Could you check a few things on this model? Use its own coordinates, in mm. Give positions to 0.01 mm unless a question says otherwise; leave off trailing zeros. Loops run counter-clockwise (first coordinate to the right, second up) from the corner with the lowest first, then second, coordinate; pieces in that order, holes last. Notation, with made-up numbers: (84, 84.25) - (94, 84.25) arc R20 cw to (94, 122.25) - close; hole circle Ø10 at (2, 77.5). An arc over 180 degrees is marked (long way). Answer in a Markdown table with one row per item. Add a question column.
```python
from build123d import *

# Parameters (mm, degrees)
SKETCH1_W           = 185
SKETCH1_H           = 84
SKETCH1_R           = 2.25
BOSS_EXTRUDE1_DEPTH = 5
SKETCH2_W           = 185
SKETCH2_H           = 79
SKETCH2_R           = 2.25
BOSS_EXTRUDE2_DEPTH = 3
CHAMFER1_SIZE       = 8
CHAMFER3_SIZE       = 3
SKETCH3_W           = 7.071067812
SKETCH3_H           = 2.6
CUT_EXTRUDE1_DEPTH  = 221.270985121
SKETCH4_R           = 29
SKETCH4_R_2         = 1.75
CUT_EXTRUDE2_DEPTH  = 204.334699449


with BuildPart() as part:
    # Sketch1 → Boss-Extrude1 (new body)
    with BuildSketch(Plane.XY):
        with Locations((92.5, 42)):
            Rectangle(SKETCH1_W, SKETCH1_H)
        with Locations((15, 9)):
            Circle(SKETCH1_R, mode=Mode.SUBTRACT)
        with Locations(Location((170, 9, 0), (0, 0, 180))):
            Circle(SKETCH1_R, mode=Mode.SUBTRACT)
        with Locations((15, 72)):
            Circle(SKETCH1_R, mode=Mode.SUBTRACT)
        with Locations(Location((170, 72, 0), (0, 0, 180))):
            Circle(SKETCH1_R, mode=Mode.SUBTRACT)
    extrude(amount=-BOSS_EXTRUDE1_DEPTH)

    # Sketch2 → Boss-Extrude2 (add)
    with BuildSketch(Plane(origin=(0, 0, -5), x_dir=(-1, 0, 0), z_dir=(0, 0, -1))):
        with Locations((-92.5, 44.5)):
            Rectangle(SKETCH2_W, SKETCH2_H)
        with Locations(Location((-15, 9, 0), (0, 0, 180))):
            Circle(SKETCH2_R, mode=Mode.SUBTRACT)
        with Locations((-170, 9)):
            Circle(SKETCH2_R, mode=Mode.SUBTRACT)
        with Locations(Location((-15, 72, 0), (0, 0, 180))):
            Circle(SKETCH2_R, mode=Mode.SUBTRACT)
        with Locations((-170, 72)):
            Circle(SKETCH2_R, mode=Mode.SUBTRACT)
    extrude(amount=BOSS_EXTRUDE2_DEPTH)

    # Chamfer1
    # the kernel refuses this chamfer: 8 mm, written as the material it takes off along each edge
    with BuildSketch(Plane(origin=(185, -15.573463904, -8), x_dir=(-0.9996219169112968, 0, -0.027495876610586296), z_dir=(0, 1, 0)), Plane(origin=(0, 104.573463904, -8), x_dir=(0.9996219169112968, 0, -0.027495876610586275), z_dir=(0, -1, 0))) as chamfer1_piece_1:
        Polygon((CHAMFER1_SIZE * 0.999621916911, CHAMFER1_SIZE * 0.0274958766106), (-CHAMFER1_SIZE * 0.0274958766106, CHAMFER1_SIZE * 0.999621916911), (0, 0), align=None)
    extrude(amount=120.146927807, mode=Mode.SUBTRACT)

    # Chamfer3
    chamfer3_edges = [part.edges().sort_by_distance(p)[0] for p in [
        (92.5, 84, -8),
    ]]
    chamfer(chamfer3_edges, length=CHAMFER3_SIZE)

    # Sketch3 → Cut-Extrude1 (cut, through all, along a direction that is not the sketch's normal)
    with BuildSketch(Plane(origin=(92.5, 0, -92.5), x_dir=(-0.7071067811865452, 0, -0.7071067811865498), z_dir=(0.7071067811865498, 0, -0.7071067811865452))):
        with Locations((-127.279220614, 1.3)):
            Rectangle(SKETCH3_W, SKETCH3_H)
    extrude(amount=-CUT_EXTRUDE1_DEPTH, dir=(1, 0, 0), mode=Mode.SUBTRACT)

    # Sketch4 → Cut-Extrude2 (cut, through all)
    with BuildSketch(Plane.XY):
        with Locations((127, 50)):
            Circle(SKETCH4_R)
        with Locations((102, 74)):
            Circle(SKETCH4_R_2)
        with Locations((152, 74)):
            Circle(SKETCH4_R_2)
        with Locations((152, 24)):
            Circle(SKETCH4_R_2)
        with Locations((102, 24)):
            Circle(SKETCH4_R_2)
    extrude(amount=-CUT_EXTRUDE2_DEPTH, mode=Mode.SUBTRACT)


solid = part.part
```
(1) I want a section at A-A on x = 15. Please give me the cut outline in (y, z), then the cut area to 4 significant figures.
(2) I want a section at C-C on y = 9. Please give me the cut outline in (x, z).
(3) For pin 1 Ø1.2 at (x, y) = (97, 3.5) entering from -Z; pin 2 Ø2 at (y, z) = (43.5, -2.5) entering from -X, each with a flat end and sliding along its axis, tell me the tip position at first contact or that it passes through.
(4) We'd pull the mould along Y, two halves only. Please class faces 1 (the cylindrical face through (101.62, 72.29, -3.94)), 2 (the flat face through (94, 84, -2)), 3 (the flat face through (181, 43, -4)), 4 (the cylindrical face through (153.617, 73.33, -3.944)): pulls with the +Y half, pulls with the -Y half, needs draft (parallel to the pull), parting line crosses it, or undercut.
(5) I want a section at B-B on x = 127. Please give me the cut outline in (y, z), then the cut area to 4 significant figures.
(6) Please list where these lines run through material, in increasing order: line 1 (Y direction, x = 17, z = -7.5); line 2 (Y direction, x = 15, z = -6); line 3 (Y direction, x = 152, z = -3.5).
(7) I want a section at D-D on y = 50. Please give me the cut outline in (x, z).
Reported:
| question | item | result |
|---|---|---|
| 1 | outline | (2.6, -5) - (5, -5) - (5, -8) - (6.75, -8) - (6.75, 0) - (2.6, 0) - close; (11.25, -8) - (69.75, -8) - (69.75, 0) - (11.25, 0) - close; (74.25, -8) - (81, -8) - (84, -5) - (84, 0) - (74.25, 0) - close |
| 1 | area | 567.5 mm² |
| 2 | outline | (0, 0) - (8, -8) - (12.75, -8) - (12.75, 0) - close; (17.25, -8) - (167.75, -8) - (167.75, 0) - (17.25, 0) - close; (172.25, -8) - (177, -8) - (185, 0) - (172.25, 0) - close |
| 3 | pin 1 | z = -5 |
| 3 | pin 2 | x = 1.5 |
| 4 | face 1 | undercut |
| 4 | face 2 | pulls with the +Y half |
| 4 | face 3 | needs draft |
| 4 | face 4 | undercut |
| 5 | outline | (2.6, -5) - (5, -5) - (5, -8) - (21, -8) - (21, 0) - (2.6, 0) - close; (79, -8) - (81, -8) - (84, -5) - (84, 0) - (79, 0) - close |
| 5 | area | 175.5 mm² |
| 6 | line 1 | 5 to 7.97, 10.03 to 70.97, 73.03 to 81.5 |
| 6 | line 2 | 5 to 6.75, 11.25 to 69.75, 74.25 to 83 |
| 6 | line 3 | 2.6 to 22.25, 25.75 to 35.3, 64.7 to 72.25, 75.75 to 84 |
| 7 | outline | (0, 0) - (8, -8) - (98, -8) - (98, 0) - close; (156, -8) - (177, -8) - (185, 0) - (156, 0) - close |
